For this review, take the finished solid that the model builds, in its own axes (mm). A direction names the side the tool comes from. Give positions to 0.01 mm unless a question says otherwise; leave off trailing zeros. Loops run counter-clockwise (first coordinate to the right, second up) from the corner with the lowest first, then second, coordinate; pieces in that order, holes last. Notation, with made-up numbers: (74, 66.25) - (117, 66.25) arc R19 ccw to (117, 81.25) - close; hole circle Ø5 at (-24.5, 46.5). An arc over 180 degrees is marked (long way). Answer as CSV lines item,"result".
from build123d import *

# Parameters (mm, degrees)
ESQUISSE1_W               = 3
ESQUISSE1_H               = 8.9
T_LE_DE_BASE_PLI_E1_DEPTH = 3


# Sheet-metal steps are written as plain solids
with BuildPart() as part:
    # Esquisse1 → Tôle de base pliée1 (new body)
    with BuildSketch(Plane.XY):
        with BuildLine():
            Line((40.706473987, 1340.134366737), (89.106473987, 1340.134366737))
            Line((89.106473987, 1340.134366737), (89.106473987, 1337.234366737))
            Line((89.106473987, 1337.234366737), (92.106473987, 1337.234366737))
            Line((92.106473987, 1337.234366737), (92.106473987, 1334.434366737))
            Line((92.106473987, 1334.434366737), (89.106473987, 1334.434366737))
            Line((89.106473987, 1334.434366737), (89.106473987, 1332.434279902))
            Line((89.106473987, 1332.434279902), (86.306473987, 1332.434279902))
            Line((86.306473987, 1332.434279902), (86.306473987, 1333.734279902))
            Line((86.306473987, 1333.734279902), (83.706473987, 1333.734279902))
            Line((83.706473987, 1333.734279902), (83.706473987, 1332.434279902))
            Line((83.706473987, 1332.434279902), (79.906473987, 1332.434279902))
            Line((79.906473987, 1332.434279902), (79.906473987, 1329.234279902))
            Line((79.906473987, 1329.234279902), (83.706473987, 1329.234279902))
            Line((83.706473987, 1329.234279902), (83.706473987, 1327.934279902))
            Line((83.706473987, 1327.934279902), (86.306473987, 1327.934279902))
            Line((86.306473987, 1327.934279902), (86.306473987, 1329.234279902))
            Line((86.306473987, 1329.234279902), (89.106473987, 1329.234279902))
            Line((89.106473987, 1329.234279902), (89.106473987, 1327.234279902))
            Line((89.106473987, 1327.234279902), (92.106473987, 1327.234279902))
            Line((92.106473987, 1327.234279902), (92.106473987, 1325.034279902))
            Line((92.106473987, 1325.034279902), (89.106473987, 1325.034279902))
            Line((89.106473987, 1325.034279902), (89.106473987, 1323.534279902))
            Line((89.106473987, 1323.534279902), (92.106473987, 1323.534279902))
            Line((92.106473987, 1323.534279902), (92.106473987, 1321.434279902))
            Line((92.106473987, 1321.434279902), (88.10455642, 1321.434279902))
            ThreePointArc((88.10455642, 1321.434279902), (87.652661624, 1323.258995148), (86.401432588, 1324.661927983))
            ThreePointArc((86.401432588, 1324.661927983), (82.105492294, 1325.990171363), (77.809552, 1324.661927983))
            ThreePointArc((77.809552, 1324.661927983), (76.558356626, 1323.259032892), (76.106473987, 1321.434366737))
            Line((76.106473987, 1321.434366737), (57.706473987, 1321.434366737))
            ThreePointArc((57.706473987, 1321.434366737), (57.366344351, 1322.959443215), (56.410421102, 1324.195467962))
            ThreePointArc((56.410421102, 1324.195467962), (51.279943841, 1326.048095935), (46.149466581, 1324.195467962))
            ThreePointArc((46.149466581, 1324.195467962), (45.158922245, 1322.914677571), (44.806473987, 1321.334366737))
            Line((44.806473987, 1321.334366737), (40.706473987, 1321.334366737))
            Line((40.706473987, 1321.334366737), (40.706473987, 1323.534366737))
            Line((40.706473987, 1323.534366737), (43.706473987, 1323.534366737))
            Line((43.706473987, 1323.534366737), (43.706473987, 1325.034366737))
            Line((43.706473987, 1325.034366737), (40.706473987, 1325.034366737))
            Line((40.706473987, 1325.034366737), (40.706473987, 1327.134366737))
            Line((40.706473987, 1327.134366737), (43.706473987, 1327.134366737))
            Line((43.706473987, 1327.134366737), (43.706473987, 1329.134366737))
            Line((43.706473987, 1329.134366737), (47.506473987, 1329.134366737))
            Line((47.506473987, 1329.134366737), (47.506473987, 1327.834366737))
            Line((47.506473987, 1327.834366737), (50.106473987, 1327.834366737))
            Line((50.106473987, 1327.834366737), (50.106473987, 1329.134366737))
            Line((50.106473987, 1329.134366737), (53.856473987, 1329.134366737))
            Line((53.856473987, 1329.134366737), (53.856473987, 1332.334366737))
            Line((53.856473987, 1332.334366737), (50.106473987, 1332.334366737))
            Line((50.106473987, 1332.334366737), (50.106473987, 1333.634366737))
            Line((50.106473987, 1333.634366737), (47.506473987, 1333.634366737))
            Line((47.506473987, 1333.634366737), (47.506473987, 1332.334366737))
            Line((47.506473987, 1332.334366737), (43.706473987, 1332.334366737))
            Line((43.706473987, 1332.334366737), (43.706473987, 1336.034366737))
            Line((43.706473987, 1336.034366737), (40.706473987, 1336.034366737))
            Line((40.706473987, 1336.034366737), (40.706473987, 1340.134366737))
        make_face()
        with Locations((64.306473987, 1330.284366737)):
            Rectangle(ESQUISSE1_W, ESQUISSE1_H, mode=Mode.SUBTRACT)
    extrude(amount=-T_LE_DE_BASE_PLI_E1_DEPTH)


solid = part.part
1) Machinability: for faces 4 (the flat face through (46, 1329.134, -1)), 5 (the flat face through (62.806, 1330, -1)), 6 (the cylindrical face through (45.17, 1322.94, -1.48)), which of the approach directions +Z, -Z, +X, -X, +Y, -Y give a long, thin tool a straight path to every point of the face, cutting with its end or side? Answer none if there is none.
From the geometry:
face 4,"+Z, -Z, -X"
face 5,"+Z, -Z"
face 6,"+Z, -Z, -Y"
2) Wall thickness on line 1 (X direction, y = 1326.75, z = -1.1); line 2 (X direction, y = 1324, z = -1.8) (3 decimals); line 3 (X direction, y = 1333.25, z = -0.9): over which ranges is each line inside the solid? List them lowest first. Write a range as from..to.
From the geometry:
line 1,"x = 40.71..62.81, 65.81..92.11"
line 2,"x = 43.706..45.932, 56.627..77.066, 87.145..89.106"
line 3,"x = 43.71..47.51, 50.11..62.81, 65.81..83.71, 86.31..89.11"
3) Consider section A-A on x = 65. Write out the cut boundary in (y, z).
From the geometry:
outline,"(1321.43, -3) - (1325.83, -3) - (1325.83, 0) - (1321.43, 0) - close; (1334.73, -3) - (1340.13, -3) - (1340.13, 0) - (1334.73, 0) - close"
4) Draft analysis for pull direction Y (two halves, no side actions). For faces 1 (the flat face through (42, 1325.034, -1)), 2 (the flat face through (40.706, 1326, -1)), 3 (the cylindrical face through (87.665, 1323.235, -1.479)), state which applies: pulls with the +Y half, pulls with the -Y half, needs draft (parallel to the pull), parting line crosses it, or undercut.
From the geometry:
face 1,"undercut"
face 2,"needs draft"
face 3,"pulls with the -Y half"
5) Insertion check: P1, Ø0.8, axis at y = 1324, z = -1.5, coming from the -X side; P2, Ø0.6, axis at y = 1333, z = -1, coming from the +X side; P3, Ø1, axis at x = 83.5, z = -1, coming from the -Y side. Each pin has a flat end and moves straight along its axis. Give the tip position at first contact, or say it passes through.
From the geometry:
P1,"stops at x = 43.71"
P2,"stops at x = 89.11"
P3,"stops at y = 1325.75"
6) Consider section B-B on x = 52.5. Write out the cut boundary in (y, z).
From the geometry:
outline,"(1325.95, -3) - (1329.13, -3) - (1329.13, 0) - (1325.95, 0) - close; (1332.33, -3) - (1340.13, -3) - (1340.13, 0) - (1332.33, 0) - close"
